```python
from build123d import *

# Parameters (mm, degrees)
F3_DEPTH = 3.175
F4_SIZE  = 0.762
F5_R     = 0.381
F6_R     = 0.381


with BuildPart() as f1:
    # F0 (on Front) → F1 (revolve)
    with BuildSketch(Plane.XZ):
        Polygon((-24.60625, 0), (0, 0), (0, 6.223), (-3.175, 6.223), (-3.175, 3.937), (-15.08125, 3.937), (-15.08125, 2.286), (-15.84325, 2.286), (-18.1112926098, 3.1115), (-24.60625, 3.1115), align=None)
    revolve(axis=Axis((2.7985820894, 0, 0), (1, 0, 0)))

    # F2 (on face) → F3 (cut, through all)
    with BuildSketch(Plane.YZ):
        with BuildLine():
            Line((-5.2128290459, 3.3988442651), (-0.3370709541, 6.2138645119))
            ThreePointArc((-0.3370709541, 6.2138645119), (-3.1115, 5.3892760878), (-5.2128290459, 3.3988442651))
        make_face()
        with BuildLine():
            ThreePointArc((5.2128290459, 3.3988442651), (3.1115, 5.3892760878), (0.3370709541, 6.2138645119))
            Line((0.3370709541, 6.2138645119), (5.2128290459, 3.3988442651))
        make_face()
        with BuildLine():
            ThreePointArc((6.223, 0), (6.0523861699, 1.447187151), (5.5499, 2.8150202468))
            Line((5.5499, 2.8150202468), (5.5499, -2.8150202468))
            ThreePointArc((5.5499, -2.8150202468), (6.0523861699, -1.447187151), (6.223, 0))
        make_face()
        with BuildLine():
            ThreePointArc((0.3370709541, -6.2138645119), (3.1115, -5.3892760878), (5.2128290459, -3.3988442651))
            Line((5.2128290459, -3.3988442651), (0.3370709541, -6.2138645119))
        make_face()
        with BuildLine():
            Line((-0.3370709541, -6.2138645119), (-5.2128290459, -3.3988442651))
            ThreePointArc((-5.2128290459, -3.3988442651), (-3.1115, -5.3892760878), (-0.3370709541, -6.2138645119))
        make_face()
        with BuildLine():
            Line((-5.5499, -2.8150202468), (-5.5499, 2.8150202468))
            ThreePointArc((-5.5499, 2.8150202468), (-6.223, 0), (-5.5499, -2.8150202468))
        make_face()
    extrude(amount=-F3_DEPTH, mode=Mode.SUBTRACT)

    # F4
    f4_edges = [f1.edges().sort_by_distance(p)[0] for p in [
        (-24.60625, 0, -3.1115),
    ]]
    chamfer(f4_edges, length=F4_SIZE)

    # F5
    f5_edges = [f1.edges().sort_by_distance(p)[0] for p in [
        (-3.175, 0, -3.937),
    ]]
    fillet(f5_edges, radius=F5_R)

    # F6
    f6_edges = [f1.edges().sort_by_distance(p)[0] for p in [
        (-15.08125, 0, -2.286),
    ]]
    fillet(f6_edges, radius=F6_R)


solid = f1.part
```
CAD build for the part. Positions are in the model's coordinates, mm. A direction names the side the tool comes from. Give positions to 0.01 mm unless a question says otherwise; leave off trailing zeros. Order: outer loops, then holes, each group sorted by start corner. A loop starts at its lowest first (then second) coordinate and runs counter-clockwise, first axis right, second up.
(1) Mould opens along X. For faces 4 (the flat face through (0, 0, 0)), 5 (the flat face through (-15.081, 3, 1)), 6 (the flat face through (-1.565, 2.809, -4.787)) say: released by +X, released by -X, zero draft, split by the parting line, or undercut.
(2) Tool access for faces 1 (the cylindrical face through (-21.02, 3.04, -0.67)), 2 (the flat face through (-1.565, -2.741, -4.826)), 3 (the conical face through (-16.24, -0.73, 2.32)): list every direction of +Z, -Z, +X, -X, +Y, -Y with a clear straight run to the whole face (end or side of a thin tool).
(3) Drill centre lines: L1, parallel to X at y = 3.25, z = -1.5; L2, parallel to X at y = -3.5, z = -3.25 (3 decimals); L3, parallel to Y at x = -16, z = -0.5. Where is each one in solid material? Low to high.
(4) Saw through at C-C, the plane x = -22.5. Give the cut face in (y, z).
(5) Flat gauge pins, fed straight in: pin 1 (3 mm diameter, centred on x = -12.5, z = 3, fed in from +Y); pin 2 (4 mm diameter, centred on x = -10, y = 4, fed in from +Z); pin 3 (6 mm diameter, centred on x = -20, y = 4, fed in from -Z). Where does each tip first touch, or does it go through?
Results found:
1. face 4: released by +X
1. face 5: undercut
1. face 6: zero draft
2. face 1: -X
2. face 2: -Z, +X, -X, -Y
2. face 3: none
3. L1: x = -15.08 to 0
3. L2: x = -3.175 to 0
3. L3: y = -2.29 to 2.29
4. outline: circle Ø6.22 at (0, 0)
5. pin 1: stops at y = 3.64
5. pin 2: stops at z = 3.39
5. pin 3: stops at z = -2.95
